Read the model definition and answer for the solid it produces. Units are mm, in the model's axes. Round coordinates to 2 decimals unless told otherwise and drop trailing zeros. Write each loop counter-clockwise with the first axis right and the second up, starting at its lowest first coordinate (ties: lowest second). Pieces come first, ordered by that corner, then holes. Notation, with made-up numbers: M 58.5,24.5 L 84.5,24.5 A24 ccw 84.5,46.5 Z; hole C 34,-7 d2. An arc over 180 degrees is marked long. Use one line per item in the form item = value. Start each with the question number.
```python
from build123d import *

# Parameters (mm, degrees)
F0_R     = 1.5
F0_W     = 40
F0_H     = 6.7
F0_H_2   = 1.6
F0_W_2   = 10
F0_H_3   = 91.46
F0_W_3   = 15
F0_H_4   = 1.7
F0_H_5   = 15
F0_H_6   = 5
F0_H_7   = 52.41
F0_H_8   = 3.65
F0_H_9   = 1.48
F0_W_4   = 3
F0_H_10  = 0.6
F0_H_11  = 1.4
F1_DEPTH = 2.9972


# Not quite as in the source:
# - a feature names something its author has since deleted; it is built from what else it names


with BuildPart() as f1:
    # F0 (on Front) → F1 (new body)
    with BuildSketch(Plane.XZ):
        with BuildLine():
            Line((-24.4680281997, 132.5136111658), (-91.7680281997, 132.5136111658))
            ThreePointArc((-91.7680281997, 132.5136111658), (-95.3035621056, 131.0491450717), (-96.7680281997, 127.5136111658))
            Line((-96.7680281997, 127.5136111658), (-96.7680281997, -22.4863888342))
            Line((-96.7680281997, -22.4863888342), (-86.7680281997, -22.4863888342))
            Line((-86.7680281997, -22.4863888342), (-86.7680281997, -1.5222273069))
            Line((-86.7680281997, -1.5222273069), (-86.7680281997, 0))
            Line((-86.7680281997, 0), (-86.7680281997, 16.1536111658))
            Line((-86.7680281997, 16.1536111658), (-86.7680281997, 20.4536111658))
            Line((-86.7680281997, 20.4536111658), (-86.7680281997, 21.4536111658))
            Line((-86.7680281997, 21.4536111658), (-89.7680281997, 21.4536111658))
            Line((-89.7680281997, 21.4536111658), (-89.7680281997, 22.0536111658))
            Line((-89.7680281997, 22.0536111658), (-89.7680281997, 22.8536111658))
            Line((-89.7680281997, 22.8536111658), (-89.7680281997, 23.4536111658))
            Line((-89.7680281997, 23.4536111658), (-86.7680281997, 23.4536111658))
            Line((-86.7680281997, 23.4536111658), (-86.7680281997, 24.4536111658))
            Line((-86.7680281997, 24.4536111658), (-86.7680281997, 24.6436111658))
            Line((-86.7680281997, 24.6436111658), (-86.7680281997, 53.4536111658))
            Line((-86.7680281997, 53.4536111658), (-86.7680281997, 56.4536111658))
            Line((-86.7680281997, 56.4536111658), (-86.7680281997, 60.7536111658))
            Line((-86.7680281997, 60.7536111658), (-86.7680281997, 61.4536111658))
            Line((-86.7680281997, 61.4536111658), (-86.7680281997, 122.5136111658))
            Line((-86.7680281997, 122.5136111658), (-40.4680281997, 122.5136111658))
            Line((-40.4680281997, 122.5136111658), (-39.4680281997, 122.5136111658))
            Line((-39.4680281997, 122.5136111658), (-39.4680281997, 124.2136111658))
            Line((-39.4680281997, 124.2136111658), (-49.4680281997, 124.2136111658))
            Line((-49.4680281997, 124.2136111658), (-49.4680281997, 125.8136111658))
            Line((-49.4680281997, 125.8136111658), (-28.7680281997, 125.8136111658))
            Line((-28.7680281997, 125.8136111658), (-24.4680281997, 125.8136111658))
            Line((-24.4680281997, 125.8136111658), (-24.4680281997, 132.5136111658))
        make_face()
        with Locations((-91.7680281997, -17.4863888342)):
            Circle(F0_R, mode=Mode.SUBTRACT)
        with Locations((-91.7680281997, 127.5136111658)):
            Circle(F0_R, mode=Mode.SUBTRACT)
        with Locations((-4.4680281997, 129.1636111658)):
            Rectangle(F0_W, F0_H)
        with BuildLine():
            Line((82.8319718003, 132.5136111658), (15.5319718003, 132.5136111658))
            Line((15.5319718003, 132.5136111658), (15.5319718003, 125.8136111658))
            Line((15.5319718003, 125.8136111658), (21.2319718003, 125.8136111658))
            Line((21.2319718003, 125.8136111658), (40.5319718003, 125.8136111658))
            Line((40.5319718003, 125.8136111658), (40.5319718003, 124.2136111658))
            Line((40.5319718003, 124.2136111658), (30.5319718003, 124.2136111658))
            Line((30.5319718003, 124.2136111658), (30.5319718003, 122.5136111658))
            Line((30.5319718003, 122.5136111658), (40.5319718003, 122.5136111658))
            Line((40.5319718003, 122.5136111658), (77.8319718003, 122.5136111658))
            Line((77.8319718003, 122.5136111658), (77.8319718003, 61.4536111658))
            Line((77.8319718003, 61.4536111658), (77.8319718003, 60.7536111658))
            Line((77.8319718003, 60.7536111658), (77.8319718003, 56.4536111658))
            Line((77.8319718003, 56.4536111658), (77.8319718003, 53.4536111658))
            Line((77.8319718003, 53.4536111658), (77.8319718003, 24.6436111658))
            Line((77.8319718003, 24.6436111658), (77.8319718003, 24.4536111658))
            Line((77.8319718003, 24.4536111658), (77.8319718003, 23.4536111658))
            Line((77.8319718003, 23.4536111658), (80.8319718003, 23.4536111658))
            Line((80.8319718003, 23.4536111658), (80.8319718003, 22.8536111658))
            Line((80.8319718003, 22.8536111658), (80.8319718003, 21.4536111658))
            Line((80.8319718003, 21.4536111658), (77.8319718003, 21.4536111658))
            Line((77.8319718003, 21.4536111658), (77.8319718003, 20.4536111658))
            Line((77.8319718003, 20.4536111658), (77.8319718003, 16.1536111658))
            Line((77.8319718003, 16.1536111658), (77.8319718003, 4.5))
            Line((77.8319718003, 4.5), (77.8319718003, -1.5222273069))
            Line((77.8319718003, -1.5222273069), (77.8319718003, -128.9463888342))
            Line((77.8319718003, -128.9463888342), (1.2319718003, -128.9463888342))
            Line((1.2319718003, -128.9463888342), (1.2319718003, -130.4263888342))
            Line((1.2319718003, -130.4263888342), (3.7319718003, -130.4263888342))
            Line((3.7319718003, -130.4263888342), (3.7319718003, -132.0263888342))
            Line((3.7319718003, -132.0263888342), (-11.2680281997, -132.0263888342))
            Line((-11.2680281997, -132.0263888342), (-11.2680281997, -130.4263888342))
            Line((-11.2680281997, -130.4263888342), (-8.7680281997, -130.4263888342))
            Line((-8.7680281997, -130.4263888342), (-8.7680281997, -128.9463888342))
            Line((-8.7680281997, -128.9463888342), (-86.7680281997, -128.9463888342))
            Line((-86.7680281997, -128.9463888342), (-96.7680281997, -128.9463888342))
            Line((-96.7680281997, -128.9463888342), (-96.7680281997, -132.2803888342))
            Line((-96.7680281997, -132.2803888342), (-96.7680281997, -133.9463888342))
            ThreePointArc((-96.7680281997, -133.9463888342), (-95.3035621056, -137.4819227401), (-91.7680281997, -138.9463888342))
            Line((-91.7680281997, -138.9463888342), (82.8319718003, -138.9463888342))
            ThreePointArc((82.8319718003, -138.9463888342), (86.3675057063, -137.4819227401), (87.8319718003, -133.9463888342))
            Line((87.8319718003, -133.9463888342), (87.8319718003, 127.5136111658))
            ThreePointArc((87.8319718003, 127.5136111658), (86.3675057063, 131.0491450717), (82.8319718003, 132.5136111658))
        make_face()
        with Locations((82.8319718003, -133.9463888342)):
            Circle(F0_R, mode=Mode.SUBTRACT)
        with Locations((82.8319718003, -17.4863888342)):
            Circle(F0_R, mode=Mode.SUBTRACT)
        with Locations((82.8319718003, 127.5136111658)):
            Circle(F0_R, mode=Mode.SUBTRACT)
        Polygon((-24.4680281997, 124.2136111658), (-24.4680281997, 125.8136111658), (-28.7680281997, 125.8136111658), (-49.4680281997, 125.8136111658), (-49.4680281997, 124.2136111658), (-39.4680281997, 124.2136111658), align=None)
        with Locations((-4.4680281997, 125.0136111658)):
            Rectangle(F0_W, F0_H_2)
        with Locations((-91.7680281997, -68.2163888342)):
            Rectangle(F0_W_2, F0_H_3)
        Polygon((21.2319718003, 125.8136111658), (15.5319718003, 125.8136111658), (15.5319718003, 124.2136111658), (30.5319718003, 124.2136111658), (40.5319718003, 124.2136111658), (40.5319718003, 125.8136111658), align=None)
        with Locations((-31.9680281997, 123.3636111658)):
            Rectangle(F0_W_3, F0_H_4)
        with Locations((-4.4680281997, 123.3636111658)):
            Rectangle(F0_W, F0_H_4)
        with Locations((-91.7680281997, -121.4463888342)):
            Rectangle(F0_W_2, F0_H_5)
        with Locations((-91.7680281997, -118.9463888342)):
            Circle(F0_R, mode=Mode.SUBTRACT)
        Polygon((-86.7680281997, -1.5222273069), (-86.7680281997, -22.4863888342), (-86.7680281997, -113.9463888342), (-86.7680281997, -128.9463888342), (-8.7680281997, -128.9463888342), (1.2319718003, -128.9463888342), (77.8319718003, -128.9463888342), (77.8319718003, -1.5222273069), align=None)
        with Locations((23.0319718003, 123.3636111658)):
            Rectangle(F0_W_3, F0_H_4)
        with Locations((-31.9680281997, 120.0136111658)):
            Rectangle(F0_W_3, F0_H_6)
        with Locations((-4.4680281997, 120.0136111658)):
            Rectangle(F0_W, F0_H_6)
        with Locations((23.0319718003, 120.0136111658)):
            Rectangle(F0_W_3, F0_H_6)
        Polygon((-39.4680281997, 117.5136111658), (-39.4680281997, 122.5136111658), (-40.4680281997, 122.5136111658), (-86.7680281997, 122.5136111658), (-86.7680281997, 61.4536111658), (-79.4680281997, 61.4536111658), (-79.4680281997, 65.1036111658), (-66.1611799171, 65.1036111658), align=None)
        with Locations((-63.7680281997, 79.6436111658)):
            Circle(F0_R, mode=Mode.SUBTRACT)
        Polygon((-24.4680281997, 65.1036111658), (-24.4680281997, 117.5136111658), (-39.4680281997, 117.5136111658), (-66.1611799171, 65.1036111658), align=None)
        with Locations((-4.4680281997, 91.3086111658)):
            Rectangle(F0_W, F0_H_7)
        Polygon((40.5319718003, 122.5136111658), (30.5319718003, 122.5136111658), (30.5319718003, 117.5136111658), (57.2251235178, 65.1036111658), (70.5319718003, 65.1036111658), (70.5319718003, 61.4536111658), (77.8319718003, 61.4536111658), (77.8319718003, 122.5136111658), align=None)
        with Locations((54.8319718003, 79.6436111658)):
            Circle(F0_R, mode=Mode.SUBTRACT)
        Polygon((30.5319718003, 117.5136111658), (15.5319718003, 117.5136111658), (15.5319718003, 65.1036111658), (57.2251235178, 65.1036111658), align=None)
        with Locations((-4.4680281997, 63.2786111658)):
            Rectangle(F0_W, F0_H_8)
        Polygon((-24.4680281997, 61.4536111658), (-24.4680281997, 65.1036111658), (-66.1611799171, 65.1036111658), (-68.0201763638, 61.4536111658), align=None)
        with Locations((-3.7680281997, -129.6863888342)):
            Rectangle(F0_W_2, F0_H_9)
        Polygon((57.2251235178, 65.1036111658), (15.5319718003, 65.1036111658), (15.5319718003, 61.4536111658), (59.0841199644, 61.4536111658), align=None)
        Polygon((-68.0201763638, 61.4536111658), (-66.1611799171, 65.1036111658), (-79.4680281997, 65.1036111658), (-79.4680281997, 61.4536111658), align=None)
        Polygon((1.2319718003, -130.4263888342), (-8.7680281997, -130.4263888342), (-11.2680281997, -130.4263888342), (-11.2680281997, -132.0263888342), (3.7319718003, -132.0263888342), (3.7319718003, -130.4263888342), align=None)
        Polygon((70.5319718003, 65.1036111658), (57.2251235178, 65.1036111658), (59.0841199644, 61.4536111658), (70.5319718003, 61.4536111658), align=None)
        Polygon((-89.7680281997, 21.4536111658), (-86.7680281997, 21.4536111658), (-86.7680281997, 22.8536111658), (-89.7680281997, 22.8536111658), (-89.7680281997, 22.0536111658), align=None)
        with Locations((-88.2680281997, 23.1536111658)):
            Rectangle(F0_W_4, F0_H_10)
        with Locations((79.3319718003, 22.1536111658)):
            Rectangle(F0_W_4, F0_H_11)
        with Locations((79.3319718003, 23.1536111658)):
            Rectangle(F0_W_4, F0_H_10)
    extrude(amount=F1_DEPTH)


solid = f1.part
```
Q1. Find section C-C on y = -1.1. Count the separate pieces of the cut face and the enclosed holes in it, and give its area (3 significant figures).
Q2. Straight lines are drawn through the part: line 1 (Z direction, x = 54.5, y = -0.9); line 2 (X direction, y = -1.05, z = 48.5); line 3 (Z direction, x = 30, y = -1.45). For each, find the intervals that lie inside material, in ascending order. Write a range as [from, to].
Q3. This flat-tipped pin is pushed along its axis until it touches: pin 1 Ø4 at (x, z) = (82.83, -17.49) entering from +Y. Where does it stop, or does it pass through?
Q4. Find section B-B on x = -33. Write down the section's boundary in (y, z), and give its area (3 significant figures).
Q5. Find section A-A on z = 42.5. Write down the section's boundary in (x, y).
Response:
q1.separate_pieces = 1
q1.enclosed_holes = 9
q1.area = 39,700 mm²
q2.line_1 = [-138.95, -1.52], [61.45, 78.18], [81.11, 132.51]
q2.line_2 = [-96.77, -86.77], [77.83, 87.83]
q2.line_3 = [-138.95, -1.52], [61.45, 132.51]
q3.pin_1 = 0
q4.outline = M -3,-138.95 L 0,-138.95 L 0,-1.52 L -3,-1.52 Z; M -3,61.45 L 0,61.45 L 0,132.51 L -3,132.51 Z
q4.area = 625 mm²
q5.outline = M -96.77,-3 L -86.77,-3 L -86.77,0 L -96.77,0 Z; M 77.83,-3 L 87.83,-3 L 87.83,0 L 77.83,0 Z
